from build123d import *

# Parameters (mm, degrees)
F0_R     = 6.35
F1_DEPTH = 6.35


with BuildPart() as f1:
    # F0 (on Front) → F1 (new body, symmetric)
    with BuildSketch(Plane.XZ):
        with BuildLine():
            Line((101.6, 19.05), (0, 19.05))
            ThreePointArc((0, 19.05), (-19.05, 0), (0, -19.05))
            Line((0, -19.05), (101.6, -19.05))
            ThreePointArc((101.6, -19.05), (120.65, 0), (101.6, 19.05))
        make_face()
        Circle(F0_R, mode=Mode.SUBTRACT)
        with Locations((101.6, 0)):
            Circle(F0_R, mode=Mode.SUBTRACT)
    extrude(amount=F1_DEPTH, both=True)


solid = f1.part
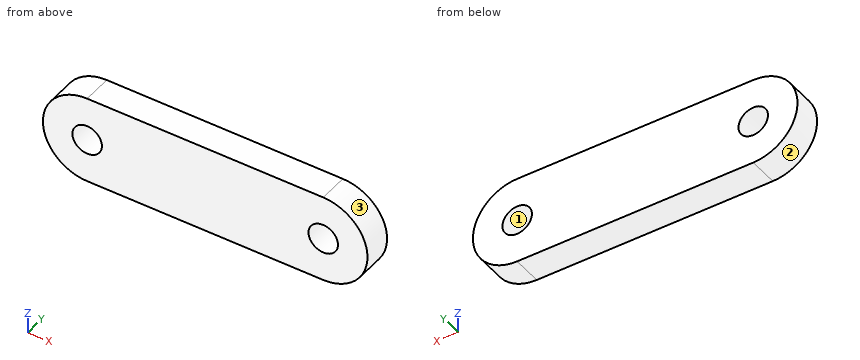
Input: part model. Units: mm. Frame: model coordinates. Face numbers are marked on the shaded views. Coordinates: 2 decimals unless noted, no trailing zeros. Order: outer loops, then holes, each group sorted by start corner. A loop starts at its lowest first (then second) coordinate and runs counter-clockwise, first axis right, second up. Notation, with made-up numbers: M 33.25,-1.75 L 57.25,-1.75 A38 ccw 57.25,36.25 Z; hole C 55.5,-9.75 d1. An arc over 180 degrees is marked long. Write item = value, one per line. Start each with the question number.
(1) Line query: line 1 along Z through (x, y) = (101.6, 2); line 2 along X through (y, z) = (4.75, 5.5); line 3 along X through (y, z) = (-1.5, -4). Output: solid intervals per line, ascending. Write a range as [from, to].
(2) Section D-D on z = 8. Output: boundary loops of the cut face in (x, y), and give its area (3 significant figures).
(3) Section C-C on y = 2.5. Output: boundary loops of the cut face in (x, z), and give its area (3 significant figures).
(4) Section A-A on z = 2. Output: boundary loops of the cut face in (x, y), and give its area (3 significant figures).
(5) First-contact query: P1, Ø1.5, axis at y = -0.5, z = -10.5, coming from the -X side; P2, Ø4, axis at y = -2, z = -8.5, coming from the +X side. Flat tips, straight axial feed; report the tip coordinate or a pass-through.
(6) Pull-direction query (X, two-part tool) for the marked faces 1, 2 and 3; classes: released by +X, released by -X, zero draft, split by the parting line, or undercut.
(7) Section B-B on x = 105.5. Output: boundary loops of the cut face in (y, z), and give its area (3 significant figures).
Result set:
q1.line_1 = [-19.05, -6.35], [6.35, 19.05]
q1.line_2 = [-18.24, -3.17], [3.17, 98.43], [104.77, 119.84]
q1.line_3 = [-18.63, -4.93], [4.93, 96.67], [106.53, 120.23]
q2.outline = M -17.29,-6.35 L 118.89,-6.35 L 118.89,6.35 L -17.29,6.35 Z
q2.area = 1,730 mm²
q3.outline = M 0,-19.05 L 101.6,-19.05 A19.05 ccw 101.6,19.05 L 0,19.05 A19.05 ccw Z; hole C 0,0 d12.7; hole C 101.6,0 d12.7
q3.area = 4,760 mm²
q4.outline = M -18.94,-6.35 L -6.03,-6.35 L -6.03,6.35 L -18.94,6.35 Z; M 6.03,-6.35 L 95.57,-6.35 L 95.57,6.35 L 6.03,6.35 Z; M 107.63,-6.35 L 120.54,-6.35 L 120.54,6.35 L 107.63,6.35 Z
q4.area = 1,470 mm²
q5.P1 = -16.37
q5.P2 = 119.51
q6.face_1 = undercut
q6.face_2 = released by -X
q6.face_3 = released by +X
q7.outline = M -6.35,-18.65 L 6.35,-18.65 L 6.35,-5.01 L -6.35,-5.01 Z; M -6.35,5.01 L 6.35,5.01 L 6.35,18.65 L -6.35,18.65 Z
q7.area = 346 mm²
